Read the model definition and answer for the solid it produces. Units are mm, in the model's axes. Round coordinates to 2 decimals unless told otherwise and drop trailing zeros. Order: outer loops, then holes, each group sorted by start corner. A loop starts at its lowest first (then second) coordinate and runs counter-clockwise, first axis right, second up. Notation, with made-up numbers: M 46.25,28 L 80.25,28 A17 ccw 80.25,49 Z; hole C 57.25,51.25 d4. An arc over 180 degrees is marked long. Answer as CSV lines item,"result".
```python
from build123d import *

# Parameters (mm, degrees)
SKETCH_1_W               = 24
SKETCH_1_H               = 8
EXTRUDE_1_DEPTH          = 250
CUT_EXTRUDE_3_DEPTH      = 251.319795462
CUT_EXTRUDE_3_DEPTH_BACK = 251.319795462
SKETCH_2_R               = 2.5


with BuildPart() as part:
    # 草图1 → 凸台-拉伸1 (new body)
    with BuildSketch(Plane(origin=(0, 0, 0), x_dir=(0, 0, -1), z_dir=(1, 0, 0))):
        Rectangle(SKETCH_1_W, SKETCH_1_H)
    extrude(amount=EXTRUDE_1_DEPTH)

    # 草图2 → 切除-拉伸3 (cut, two sides: drawn at the far end of the back side and taken through both)
    with BuildSketch(Plane(origin=(0, 0, 0), x_dir=(1, 0, 0), z_dir=(0, 1, 0)).offset(-CUT_EXTRUDE_3_DEPTH_BACK)):
        with Locations(Location((163, 0, 0), (0, 0, 270))):
            Circle(SKETCH_2_R)
        with BuildLine():
            Line((133, 2.5), (139, 2.5))
            ThreePointArc((139, 2.5), (141.5, 0), (139, -2.5))
            Line((139, -2.5), (133, -2.5))
            ThreePointArc((133, -2.5), (130.5, 0), (133, 2.5))
        make_face()
    extrude(amount=CUT_EXTRUDE_3_DEPTH + CUT_EXTRUDE_3_DEPTH_BACK, mode=Mode.SUBTRACT)


solid = part.part
```
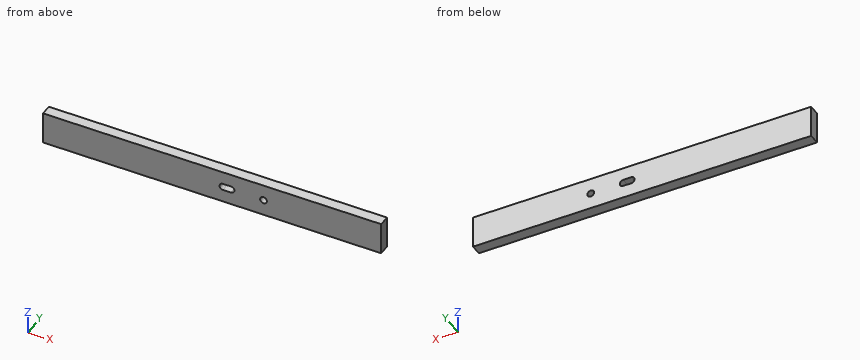
Item 1: A cutting plane is placed at A-A, the plane z = 0. Determine the outline of the cut face in (x, y).
Ans:
outline,"M 0,-4 L 130.5,-4 L 130.5,4 L 0,4 Z; M 141.5,-4 L 160.5,-4 L 160.5,4 L 141.5,4 Z; M 165.5,-4 L 250,-4 L 250,4 L 165.5,4 Z"
Item 2: Find the intervals of material crossed by probe 1 along X at (y, z) = (0, 0); probe 2 along Z at (x, y) = (163, -1); probe 3 along X at (y, z) = (2, -1.5), in increasing order. Write a range as [from, to].
Ans:
probe 1,"[0, 130.5], [141.5, 160.5], [165.5, 250]"
probe 2,"[-12, -2.5], [2.5, 12]"
probe 3,"[0, 131], [141, 161], [165, 250]"
Item 3: A cutting plane is placed at B-B, the plane x = 163. Determine the outline of the cut face in (y, z), and give its area (3 significant figures).
Ans:
outline,"M -4,-12 L 4,-12 L 4,-2.5 L -4,-2.5 Z; M -4,2.5 L 4,2.5 L 4,12 L -4,12 Z"
area,"152 mm2"
